Read the model definition and answer for the solid it produces. Units are mm, in the model's axes. A direction names the side the tool comes from. Coordinates: 2 decimals unless noted, no trailing zeros. Order: outer loops, then holes, each group sorted by start corner. A loop starts at its lowest first (then second) coordinate and runs counter-clockwise, first axis right, second up. Notation, with made-up numbers: M 4,3.25 L 19,3.25 A11 ccw 19,20.25 Z; hole C -13.5,-2.5 d10. An arc over 180 degrees is marked long. Write each question's results on one line, items separated by ' | '.
```python
from build123d import *

# Parameters (mm, degrees)
SKETCH1_W               = 80.9625
SKETCH1_H               = 57.15
BOSS_EXTRUDE1_DEPTH     = 6.35
SKETCH2_W               = 6.604
SKETCH2_H               = 25.654
CUT_EXTRUDE1_DEPTH      = 7.35
F_1_4_CLEARANCE_HOLE1_D = 6.7564
SKETCH5_W               = 4.7625
SKETCH5_H               = 47.625
BOSS_EXTRUDE3_DEPTH     = 6.35
FILLET1_R               = 3.175
SKETCH6_W               = 12.954
SKETCH6_H               = 19.304
CUT_EXTRUDE2_DEPTH      = 7.35


with BuildPart() as part:
    # Sketch1 → Boss-Extrude1 (new body)
    with BuildSketch(Plane(origin=(0, 0, 0), x_dir=(1, 0, 0), z_dir=(0, 1, 0))):
        Rectangle(SKETCH1_W, SKETCH1_H)
    extrude(amount=BOSS_EXTRUDE1_DEPTH)

    # Sketch2 → Cut-Extrude1 (cut, through all)
    with BuildSketch(Plane(origin=(0, 0, 0), x_dir=(-1, 0, 0), z_dir=(0, -1, 0))):
        with Locations((-7.14375, -1.389678771)):
            Rectangle(SKETCH2_W, SKETCH2_H)
        with Locations((18.25625, -1.389678771)):
            Rectangle(SKETCH2_W, SKETCH2_H)
    extrude(amount=-CUT_EXTRUDE1_DEPTH, mode=Mode.SUBTRACT)

    # 1/4 Clearance Hole1 (through all)
    with Locations(Plane(origin=(0, 6.35, 0), x_dir=(1, 0, 0), z_dir=(0, 1, 0))):
        with Locations((-34.13125, 19.05), (-34.13125, -19.05), (34.13125, -19.05), (34.13125, 19.05)):
            Hole(F_1_4_CLEARANCE_HOLE1_D / 2)

    # Sketch5 → Boss-Extrude3 (add)
    with BuildSketch(Plane(origin=(0, 6.35, 0), x_dir=(1, 0, 0), z_dir=(0, 1, 0))):
        with Locations((42.8625, -4.7625)):
            Rectangle(SKETCH5_W, SKETCH5_H)
        Polygon((40.48125, 28.575), (40.48125, 19.05), (45.24375, 19.05), align=None)
        with Locations((-42.8625, -4.7625)):
            Rectangle(SKETCH5_W, SKETCH5_H)
        Polygon((-40.48125, 28.575), (-45.24375, 19.05), (-40.48125, 19.05), align=None)
    extrude(amount=-BOSS_EXTRUDE3_DEPTH)

    # Fillet1
    fillet1_edges = [part.edges().sort_by_distance(p)[0] for p in [
        (-40.48125, 3.175, -28.575),
        (40.48125, 3.175, -28.575),
        (45.24375, 3.175, -19.05),
        (-45.24375, 3.175, -19.05),
    ]]
    fillet(fillet1_edges, radius=FILLET1_R)

    # Sketch6 → Cut-Extrude2 (cut, through all)
    with BuildSketch(Plane(origin=(0, 6.35, 0), x_dir=(1, 0, 0), z_dir=(0, 1, 0))):
        with Locations((-34.13125, -0.176936686)):
            Rectangle(SKETCH6_W, SKETCH6_H)
        with Locations((34.13125, -0.176936686)):
            Rectangle(SKETCH6_W, SKETCH6_H)
    extrude(amount=-CUT_EXTRUDE2_DEPTH, mode=Mode.SUBTRACT)


solid = part.part
```
(1) The part is cut by section A-A, the plane z = 19.05. Write down the section's boundary in (x, y), then the cut area to 3 significant figures.
Conclusion:
outline: M -45.24,0 L -37.51,0 L -37.51,6.35 L -45.24,6.35 Z; M -30.75,0 L 30.75,0 L 30.75,6.35 L -30.75,6.35 Z; M 37.51,0 L 45.24,0 L 45.24,6.35 L 37.51,6.35 Z | area: 489 mm²
(2) The mould has two halves that part along X. Classify faces 1 (the flat face through (-1, 6.35, 0)), 2 (the flat face through (-43.11, 3.22, -23.32)), 3 (the flat face through (7, 3, 14.217)): pulls with the +X half, pulls with the -X half, needs draft (parallel to the pull), parting line crosses it, or undercut.
Conclusion:
face 1: needs draft | face 2: pulls with the -X half | face 3: undercut
(3) The part is cut by section B-B, the plane z = 5. Write down the section's boundary in (x, y), then the cut area to 3 significant figures.
Conclusion:
outline: M -45.24,0 L -40.61,0 L -40.61,6.35 L -45.24,6.35 Z; M -27.65,0 L -21.56,0 L -21.56,6.35 L -27.65,6.35 Z; M -14.95,0 L 3.84,0 L 3.84,6.35 L -14.95,6.35 Z; M 10.45,0 L 27.65,0 L 27.65,6.35 L 10.45,6.35 Z; M 40.61,0 L 45.24,0 L 45.24,6.35 L 40.61,6.35 Z | area: 326 mm²
(4) The part is cut by section C-C, the plane y = 2.25. Count the separate pieces of the cut face and the enclosed holes in it, then the cut area to 3 significant figures.
Conclusion:
separate pieces: 1 | enclosed holes: 8 | area: 4,140 mm²
(5) The part is cut by section D-D, the plane z = 11. Write down the section's boundary in (x, y).
Conclusion:
outline: M -45.24,0 L -21.56,0 L -21.56,6.35 L -45.24,6.35 Z; M -14.95,0 L 3.84,0 L 3.84,6.35 L -14.95,6.35 Z; M 10.45,0 L 45.24,0 L 45.24,6.35 L 10.45,6.35 Z
(6) Straight lines are drawn through the part: line 1 (X direction, y = 3, z = 19.05); line 2 (X direction, y = 4, z = 3); line 3 (X direction, y = 4.5, z = -10). For each, find the intervals that lie inside material, in ascending order.
Conclusion:
line 1: -45.24 to -37.51, -30.75 to 30.75, 37.51 to 45.24 | line 2: -45.24 to -40.61, -27.65 to -21.56, -14.95 to 3.84, 10.45 to 27.65, 40.61 to 45.24 | line 3: -45.24 to -21.56, -14.95 to 3.84, 10.45 to 45.24
(7) For faces 4 (the flat face through (-1, 3, 28.575)), 5 (the flat face through (3.842, 3, 2)), determine the directions among +Z, -Z, +X, -X, +Y, -Y from which every point of the face is accessible in a straight line to the end or side of a thin tool.
Conclusion:
face 4: +Z, +X, -X, +Y, -Y | face 5: +Y, -Y
